The model under review builds one solid part; all positions refer to its coordinate system, in mm. A direction names the side the tool comes from. Round coordinates to 2 decimals unless told otherwise and drop trailing zeros. Write each loop counter-clockwise with the first axis right and the second up, starting at its lowest first coordinate (ties: lowest second). Pieces come first, ordered by that corner, then holes. Notation, with made-up numbers: (-33, -13.75) - (4, -13.75) arc R22 ccw to (4, 4.25) - close; hole circle Ø7 at (-37, 82.5). An arc over 180 degrees is marked (long way). Use one line per item in the form item = value.
from build123d import *

# Parameters (mm, degrees)
F1_DEPTH  = 16
F2_T      = -2
F3_R      = 4.5
F4_DEPTH  = 12
F6_R      = 1.35
F7_DEPTH  = 8
F8_DEPTH  = 26
F9_R      = 1.4
F9_W      = 14
F9_H      = 12
F9_R_2    = 1.5
F9_W_2    = 21
F11_DEPTH = 4
F10_R     = 1.5
F10_W     = 21
F10_H     = 12
F10_R_2   = 1.4
F12_DEPTH = 4


with BuildPart() as f1:
    # F0 (on Top) → F1 (new body)
    with BuildSketch(Plane.XY):
        with BuildLine():
            Line((-36, -67), (36, -67))
            ThreePointArc((36, -67), (39.5355339059, -65.5355339059), (41, -62))
            Line((41, -62), (41, 62))
            ThreePointArc((41, 62), (39.5355339059, 65.5355339059), (36, 67))
            Line((36, 67), (-36, 67))
            ThreePointArc((-36, 67), (-39.5355339059, 65.5355339059), (-41, 62))
            Line((-41, 62), (-41, -62))
            ThreePointArc((-41, -62), (-39.5355339059, -65.5355339059), (-36, -67))
        make_face()
    extrude(amount=F1_DEPTH)

    # F2
    f2_openings = [f1.faces().sort_by_distance(p)[0] for p in [
        (0, 0, 16),
    ]]
    offset(amount=F2_T, openings=f2_openings)

    # F3 (on face) → F4 (join)
    with BuildSketch(Plane.XY.offset(2)):
        with Locations((-23, 30)):
            Circle(F3_R)
        with Locations((-23, -30)):
            Circle(F3_R)
        with Locations((29, -30)):
            Circle(F3_R)
        with Locations((29, 30)):
            Circle(F3_R)
    extrude(amount=F4_DEPTH)

    # F6 (on mid) → F7 (cut)
    with BuildSketch(Plane.XY.offset(14)):
        with Locations((-23, 30)):
            Circle(F6_R)
        with Locations((29, 30)):
            Circle(F6_R)
        with Locations((-23, -30)):
            Circle(F6_R)
        with Locations((29, -30)):
            Circle(F6_R)
    extrude(amount=-F7_DEPTH, mode=Mode.SUBTRACT)

    # F3 (on face) → F8 (join)
    with BuildSketch(Plane.XY.offset(2)):
        with BuildLine():
            Line((-36, -65), (36, -65))
            ThreePointArc((36, -65), (38.1213203436, -64.1213203436), (39, -62))
            Line((39, -62), (39, 62))
            ThreePointArc((39, 62), (38.1213203436, 64.1213203436), (36, 65))
            Line((36, 65), (-36, 65))
            ThreePointArc((-36, 65), (-38.1213203436, 64.1213203436), (-39, 62))
            Line((-39, 62), (-39, -62))
            ThreePointArc((-39, -62), (-38.1213203436, -64.1213203436), (-36, -65))
        make_face()
        with BuildLine():
            ThreePointArc((37, -61), (36.4142135624, -62.4142135624), (35, -63))
            Line((35, -63), (-35, -63))
            ThreePointArc((-35, -63), (-36.4142135624, -62.4142135624), (-37, -61))
            Line((-37, -61), (-37, 61))
            ThreePointArc((-37, 61), (-36.4142135624, 62.4142135624), (-35, 63))
            Line((-35, 63), (35, 63))
            ThreePointArc((35, 63), (36.4142135624, 62.4142135624), (37, 61))
            Line((37, 61), (37, -61))
        make_face(mode=Mode.SUBTRACT)
    extrude(amount=F8_DEPTH)

    # F9 (on face) → F11 (cut)
    with BuildSketch(Plane(origin=(-41, 0, 0), x_dir=(0, -1, 0), z_dir=(-1, 0, 0))):
        with Locations((-13, 10)):
            Circle(F9_R)
        with Locations((13, 10)):
            Circle(F9_R)
        with Locations((0, 10)):
            Rectangle(F9_W, F9_H)
        with Locations((0, 22)):
            Rectangle(F9_W, F9_H)
        with Locations((23.825, 10)):
            Circle(F9_R_2)
        with Locations((49.825, 10)):
            Circle(F9_R_2)
        with Locations((36.825, 22)):
            Rectangle(F9_W_2, F9_H)
        Polygon((47.325, 16), (26.325, 16), (28.825, 4), (44.825, 4), align=None)
        with Locations((-45, 22)):
            Circle(F9_R)
        with Locations((55, 22)):
            Circle(F9_R)
    extrude(amount=-F11_DEPTH, mode=Mode.SUBTRACT)

    # F10 (on face) → F12 (cut)
    with BuildSketch(Plane.YZ.offset(41)):
        with Locations((-13, 10)):
            Circle(F10_R)
        with Locations((13, 10)):
            Circle(F10_R)
        with Locations((0, 22)):
            Rectangle(F10_W, F10_H)
        Polygon((10.5, 16), (-10.5, 16), (-8, 4), (8, 4), align=None)
        with Locations((45, 22)):
            Circle(F10_R_2)
        with Locations((-45, 22)):
            Circle(F10_R_2)
    extrude(amount=-F12_DEPTH, mode=Mode.SUBTRACT)


solid = f1.part
(1) The part is to be moulded in two halves that separate along X. For faces 4 (the cylindrical face through (-22.38, 28.8, 10.06)), 5 (the flat face through (0, 64, 28)), 6 (the cylindrical face through (38.14, 64.1, 21.92)), 7 (the flat face through (37, 1, 3)), say which applies: +X half, -X half, draft (parallel to the pull), parting line (faces both ways), or undercut.
Geometry results:
face_4 = undercut
face_5 = draft
face_6 = +X half
face_7 = undercut
(2) Machinability: for faces 1 (the flat face through (-39, -17, 22)), 2 (the flat face through (0, 66, 16)), 3 (the flat face through (39.028, -9.268, 10.084)), which of the approach directions +Z, -Z, +X, -X, +Y, -Y give a long, thin tool a straight path to every point of the face, cutting with its end or side? Answer none if there is none.
Geometry results:
face_1 = +Z, -X, +Y, -Y
face_2 = +Z, +Y
face_3 = +Z, +X
(3) Add section A-A on y = -55. Write out the cut boundary in (x, z), then the cut area to 3 significant figures.
Geometry results:
outline = (-41, 0) - (41, 0) - (41, 16) - (39, 16) - (39, 28) - (37, 28) - (37, 2) - (-37, 2) - (-37, 20.6) - (-39, 20.6) - (-39, 16) - (-41, 16) - close; (-39, 23.4) - (-37, 23.4) - (-37, 28) - (-39, 28) - close
area = 318 mm2
(4) Insertion check: P1, Ø3, axis at x = 39.5, y = 0, coming from the +Z side; P2, Ø8, axis at y = -35.5, z = 16, coming from the -X side; P3, Ø2.5, axis at x = 29, y = -30, coming from the +Z side. Each pin has a flat end and moves straight along its axis. Give the tip position at first contact, or say it passes through.
Geometry results:
P1 = 4
P2 = -27.01
P3 = 6
(5) Add section B-B on z = 17.5. Write out the cut boundary in (x, y) (3 decimals).
Geometry results:
outline = (-39, -62) arc R3 ccw to (-36, -65) - (36, -65) arc R3 ccw to (39, -62) - (39, -10.5) - (37, -10.5) - (37, -61) arc R2 cw to (35, -63) - (-35, -63) arc R2 cw to (-37, -61) - (-37, -47.325) - (-39, -47.325) - close; (-39, -26.325) - (-37, -26.325) - (-37, -7) - (-39, -7) - close; (-39, 7) - (-37, 7) - (-37, 61) arc R2 cw to (-35, 63) - (35, 63) arc R2 cw to (37, 61) - (37, 10.5) - (39, 10.5) - (39, 62) arc R3 ccw to (36, 65) - (-36, 65) arc R3 ccw to (-39, 62) - close
(6) Add section C-C on y = 13. Write out the cut boundary in (x, z).
Geometry results:
outline = (-41, 0) - (41, 0) - (41, 8.5) - (37, 8.5) - (37, 2) - (-37, 2) - (-37, 8.6) - (-41, 8.6) - close; (-41, 11.4) - (-37, 11.4) - (-37, 28) - (-39, 28) - (-39, 16) - (-41, 16) - close; (37, 11.5) - (41, 11.5) - (41, 16) - (39, 16) - (39, 28) - (37, 28) - close
(7) To check wall thickness, follow L1, parallel to Y at x = 2.5, z = 11.75; L2, parallel to Y at x = -13, z = 18.75; L3, parallel to Z at x = 38, y = -45. State the ranges of each line that lie inside material, in increasing order.
Geometry results:
L1 = -67 to -63, 63 to 67
L2 = -65 to -63, 63 to 65
L3 = 0 to 20.6, 23.4 to 28
(8) Add section D-D on x = 19. Write out the cut boundary in (y, z).
Geometry results:
outline = (-67, 0) - (67, 0) - (67, 16) - (65, 16) - (65, 28) - (63, 28) - (63, 2) - (-63, 2) - (-63, 28) - (-65, 28) - (-65, 16) - (-67, 16) - close
